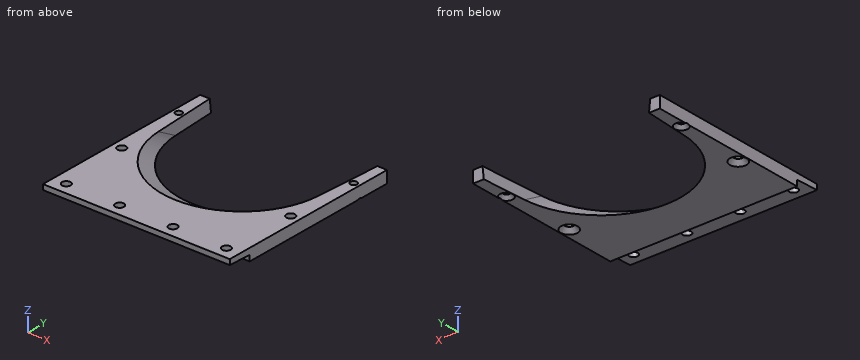
```python
from build123d import *

# Parameters (mm, degrees)
F0_W           = 200.025
F0_H           = 200.025
F1_DEPTH       = 12.7
F4_DEPTH       = 230.886
F5_R           = 4.56438
F6_DEPTH       = 25.4
F8_D           = 9.128125
F8_CSINK_D     = 17.78
F8_CSINK_ANGLE = 82
F9_D           = 7.14375
F9_CSINK_D     = 13.97
F9_CSINK_ANGLE = 82


with BuildPart() as f1:
    # F0 (on Top) → F1 (new body)
    with BuildSketch(Plane.XY):
        Rectangle(F0_W, F0_H)
    extrude(amount=F1_DEPTH)

    # F3 (on face) → F4 (cut)
    with BuildSketch(Plane(origin=(-100.0125, 0, 0), x_dir=(0, -1, 0), z_dir=(-1, 0, 0))):
        Polygon((100.0125, 0), (100.0125, 7.112), (74.6125, 6.2250124549), (74.6125, 0), align=None)
    extrude(amount=-F4_DEPTH, mode=Mode.SUBTRACT)

    # F5 (on face) → F6 (cut)
    with BuildSketch(Plane.XY.offset(12.7)):
        with Locations((-85.725, -87.3125)):
            Circle(F5_R)
        with Locations((-28.575, -87.3125)):
            Circle(F5_R)
        with Locations((28.575, -87.3125)):
            Circle(F5_R)
        with Locations((85.725, -87.3125)):
            Circle(F5_R)
    extrude(amount=-F6_DEPTH, mode=Mode.SUBTRACT)

    # F8 (through all)
    with Locations(Plane(origin=(0, 0, 0), x_dir=(1, 0, 0), z_dir=(0, 0, -1))):
        with Locations((90.4875, 11.1125), (-90.4875, 11.1125)):
            CounterSinkHole(F8_D / 2, F8_CSINK_D / 2, counter_sink_angle=F8_CSINK_ANGLE)

    # F9 (through all)
    with Locations(Plane(origin=(0, 0, 0), x_dir=(1, 0, 0), z_dir=(0, 0, -1))):
        with Locations((93.6625, -65.0875), (-93.6625, -65.0875)):
            CounterSinkHole(F9_D / 2, F9_CSINK_D / 2, counter_sink_angle=F9_CSINK_ANGLE)

    # F12: sweep along a path in F11
    with BuildLine(Plane.YZ) as f12_path:
        Line((113.8857394209, -82.55), (-216.0699394209, 107.95))
    # F10 (on face) → F12 (sweep, cut)
    with BuildSketch(Plane.XY.offset(12.7)):
        with BuildLine():
            Line((85.5720480425, 29.5142850698), (89.789, 100.0125))
            Line((89.789, 100.0125), (-89.789, 100.0125))
            Line((-89.789, 100.0125), (-85.5720480425, 29.5142850698))
            ThreePointArc((-85.5720480425, 29.5142850698), (0, -51.0921), (85.5720480425, 29.5142850698))
        make_face()
    sweep(path=f12_path.line, mode=Mode.SUBTRACT)


solid = f1.part
```
Could you check a few things on this model? Use its own coordinates, in mm. Round coordinates to 2 decimals unless told otherwise and drop trailing zeros. Put each result on its own line as item: value.
Q1. I want a section at A-A on z = 10.25. Give the number of separate pieces and of enclosed holes in the cut face, and give its area (3 significant figures).
Checks:
separate pieces: 1
enclosed holes: 8
area: 17,300 mm2
Q2. Please list where these lines run through material, in increasing order: line 1 (X direction, y = -5, z = 2); line 2 (X direction, y = 50, z = 1.5); line 3 (X direction, y = 2, z = 9). Write a range as from..to.
Checks:
line 1: -100.01..-94.2, -86.78..-62.97, 62.97..86.78, 94.2..100.01
line 2: -100.01..-85.64, 85.64..100.01
line 3: -100.01..-76.32, 76.32..100.01
Q3. For pin 1 Ø10.5 at (x, y) = (90.49, -11.11) entering from -Z; pin 2 Ø7.5 at (x, y) = (-90.49, -11.11) entering from +Z (3 decimals); pin 3 Ø10.5 at (x, y) = (-85.72, -87.31) entering from -Z, each with a flat end and sliding along its axis, tell me the tip position at first contact or that it passes through.
Checks:
pin 1: z = 4.18
pin 2: through
pin 3: z = 6.49
